Geometry: see drawing. Coordinates: mm, zero at the bounding-box minimum. Round coordinates to 2 decimals unless told otherwise and drop trailing zeros. Write each loop counter-clockwise with the first axis right and the second up, starting at its lowest first coordinate (ties: lowest second). Pieces come first, ordered by that corner, then holes.
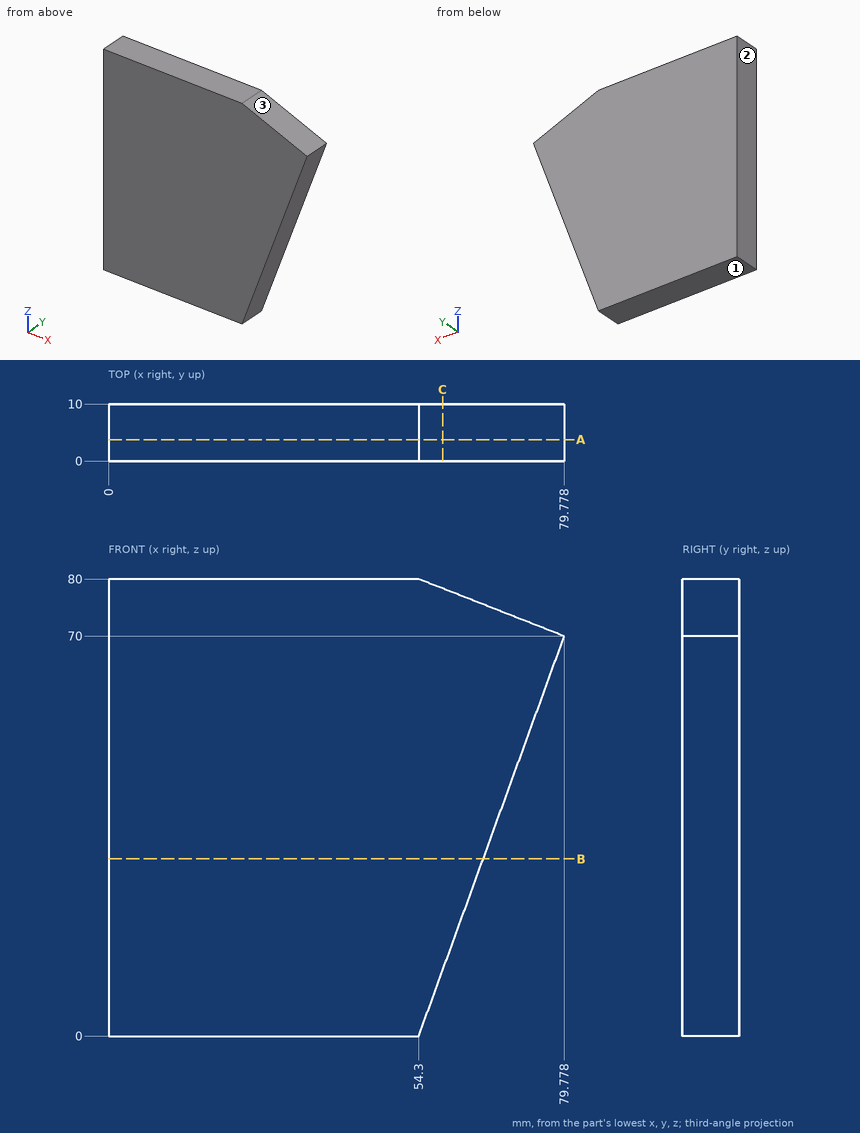
1) Section query C-C on x = 58.5. Return the cut outline in (y, z), then the cut area to 3 significant figures.
Taken from the geometry:
outline: (0, 11.54) - (10, 11.54) - (10, 78.35) - (0, 78.35) - close
area: 668 mm2
2) Material intervals for line 1 (X direction, y = 2, z = 35); line 2 (X direction, y = 7, z = 64), sorted ascending.
Taken from the geometry:
line 1: x = 0 to 67.04
line 2: x = 0 to 77.59
3) Section query B-B on z = 31. Return the cut outline in (x, y), then the cut area to 3 significant figures.
Taken from the geometry:
outline: (0, 0) - (65.58, 0) - (65.58, 10) - (0, 10) - close
area: 656 mm2
4) Section query A-A on y = 3.75. Return the cut outline in (x, z).
Taken from the geometry:
outline: (0, 0) - (54.3, 0) - (79.78, 70) - (54.3, 80) - (0, 80) - close
5) Contact query for flat-ended pins moving along their axis: P1, Ø4, axis at y = 4, z = 21, coming from the +X side; P2, Ø1, axis at y = 6.5, z = 17, coming from the +X side. Output: stop coordinate, or through.
Taken from the geometry:
P1: stops at x = 62.67
P2: stops at x = 60.67
6) Pull-direction query (X, two-part tool) for the marked faces 1, 2 and 3; classes: released by +X, released by -X, zero draft, split by the parting line, or undercut.
Taken from the geometry:
face 1: zero draft
face 2: released by -X
face 3: released by +X
